Work out the finished part from the listing and answer in its coordinate system (mm). Face numbers are marked on the shaded views. A direction names the side the tool comes from. Round coordinates to 2 decimals unless told otherwise and drop trailing zeros. Loops run counter-clockwise (first coordinate to the right, second up) from the corner with the lowest first, then second, coordinate; pieces in that order, holes last. Notation, with made-up numbers: (70, -33) -> (85, -33) arc R14 ccw to (85, -23) -> close; hole circle Ø2 at (63.5, 37). An arc over 180 degrees is marked (long way). Use CSV: the item, a comma, the result in double quotes. Start each with the question number.
Autodesk Inventor part; units mm, degrees
ref_plane "Querschnittsebene" through (-23.0321, -24.0729, 0) normal (0.8154, -0.5789, 0) x (0, 0, 1)
ref_plane "Arbeitsebene2" through (0, 8.3719, 0) normal (-1, 0, 0) x (0, 0, 1)
ref_plane "Arbeitsebene3" through (0, -70.7357, 0) normal (-0.136, 0.9907, 0) x (0, 0, 1)
sketch "Skizzenpfad" plane through (0, 0, 0) normal (0, 0, 1) x (1, 0, 0)
  arc A0 (24.2749, -23.1538) -> (-23.0321, -24.0729) centre (0, 8.3719) ccw
  arc A1 (7.4854, -36.0818) -> (5.0602, -43.6691) centre (11.756, -41.6281) ccw
  arc A2 (-11.963, -66.3767) -> (12.1791, -67.0232) centre (0, -70.7357) ccw
  arc A3 (-3.8183, -44.0246) -> (-6.3432, -35.9201) centre (-10.3952, -41.6281) ccw
  line L0 (-6.3432, -35.9201) -> (-23.0321, -24.0729)
  line L1 (24.2749, -23.1538) -> (7.4854, -36.0818)
  line L2 (5.0602, -43.6691) -> (12.1791, -67.0232)
  line L3 (-11.963, -66.3767) -> (-3.8183, -44.0246)
ref_plane "Querschnittsebene" through (-23.0321, -24.0729, 0) normal (0.8154, -0.5789, 0) x (0, 0, 1)
ref_plane "Arbeitsebene2" through (0, 8.3719, 0) normal (-1, 0, 0) x (0, 0, 1)
ref_plane "Arbeitsebene3" through (0, -70.7357, 0) normal (-0.136, 0.9907, 0) x (0, 0, 1)
sketch "Querschnitt" plane through (-23.0321, -24.0729, 0) normal (0.8154, -0.5789, 0) x (0, 0, 1)
  line L0 (-8, 0.5) -> (8, 0.5)
  line L1 (8, 0.5) -> (8, -0.5)
  line L2 (8, -0.5) -> (-8, -0.5)
  line L3 (-8, -0.5) -> (-8, 0.5)
  line L4 (-8, 0) -> (8, 0) construction
  point P0 (0, 0)
  point P1 (0, 0)
  dimension "d0" = 16
  dimension "d4" = 0.5
  dimension "d5" = 0.5
sweep "Riemen" add profiles "Querschnitt" path "Skizzenpfad"
equation "\"d0\" = da_B"
equation "\"d4\" = da_a"
equation "\"d5\" = da_a2"
equation "\"da_B\" = 16"
equation "\"da_pb\" = 5"
equation "\"da_L\" = 355"
equation "\"da_a\" = 0.5"
equation "\"da_S\" = 2.65"
equation "\"da_Beta\" = 20deg"
equation "\"da_Ht\" = 1.2"
equation "\"da_H\" = 2.2"
equation "\"da_a2\" = 0.5"
properties part number "Zahnriemen" material "Rubber"
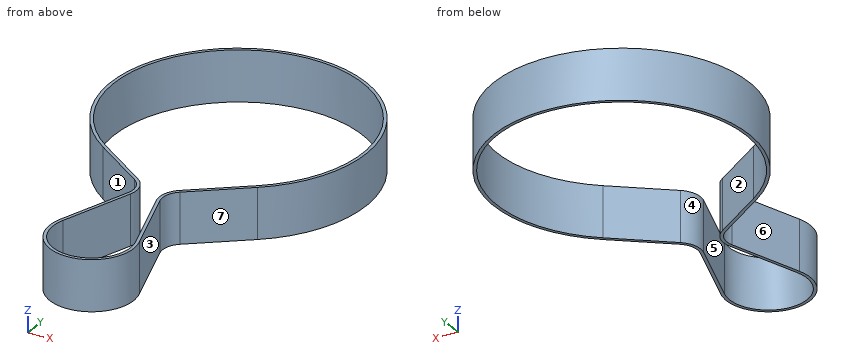
Q1. Which of the six approach directions +Z, -Z, +X, -X, +Y, -Y give full straight-line access (tool end or side, diameter ignored) to the marked faces 5, 6 and 7?
Q2. For a pull along X with two mould halves and no side action, classify the marked faces 1, 2, 3 and 4 as pulls with the +X half, pulls with the -X half, needs draft (parallel to the pull), parting line crosses it, or undercut.
Q3. Straight lines are drawn through the part: line 1 (X direction, y = 9, z = -0.25); line 2 (X direction, y = 21.5, z = 5.75); line 3 (Y direction, x = 25.5, z = 2). For each, find the intervals that lie inside material, in ascending order. Write a range as from..to.
Q4. Section B-B, the plane x = -19.5 is taken. Write down the section's boundary in (y, z).
Q5. Each of these flat-tipped pins is pushed along its axis until it touches: pin 1 (4 mm diameter, centred on x = 28, z = 3, fed in from +Y); pin 2 (2 mm diameter, centred on y = 14, z = 1.5, fed in from -X); pin 3 (3 mm diameter, centred on x = 29, z = -0.5, fed in from +Y). Where does it stop, or does it pass through?
Q6. Section C-C, the plane y = 6 is taken. Write down the section's boundary in (x, z), and give its area (3 significant figures).
Q7. Section A-A, the plane z = -2.75 is taken. Write down the section's boundary in (x, y), and give its area (3 significant figures).
Report:
1,face 5,"+Z, -Z"
1,face 6,"+Z, -Z, -X"
1,face 7,"+Z, -Z, +X"
2,face 1,"pulls with the -X half"
2,face 2,"undercut"
2,face 3,"pulls with the +X half"
2,face 4,"undercut"
3,line 1,"x = -40.28..-39.28, 39.28..40.28"
3,line 2,"x = -38.09..-37.03, 37.03..38.09"
3,line 3,"y = -22.82..-21.52, 38.26..39.56"
4,outline,"(-27.19, -8) -> (-25.97, -8) -> (-25.97, 8) -> (-27.19, 8) -> close; (42.48, -8) -> (43.63, -8) -> (43.63, 8) -> (42.48, 8) -> close"
5,pin 1,"stops at y = 39.15"
5,pin 2,"stops at x = -40.02"
5,pin 3,"stops at y = 37.82"
6,outline,"(-40.22, -8) -> (-39.22, -8) -> (-39.22, 8) -> (-40.22, 8) -> close; (39.22, -8) -> (40.22, -8) -> (40.22, 8) -> (39.22, 8) -> close"
6,area,"32.1 mm²"
7,outline,"(-23.32, -24.48) -> (-6.63, -36.33) arc R6.5 cw to (-4.29, -43.85) -> (-12.43, -66.21) arc R13.23 ccw (long way) to (12.66, -66.88) -> (5.54, -43.52) arc R6.5 cw to (7.79, -36.48) -> (24.58, -23.55) arc R40.29 ccw (long way) to start; hole (-22.74, -23.67) -> (-6.05, -35.51) arc R7.5 cw to (-3.35, -44.2) -> (-11.49, -66.55) arc R12.23 ccw (long way) to (11.7, -67.17) -> (4.58, -43.81) arc R7.5 cw to (7.18, -35.69) -> (23.97, -22.76) arc R39.29 ccw (long way) to start"
7,area,"355 mm²"
